```python
from build123d import *

# Parameters (mm, degrees)
BOSS_EXTRU_1_DEPTH      = 32
ESQUISSE1_7_R           = 15
BOSS_EXTRU_3_DEPTH      = 5
ESQUISSE1_8_R           = 21.5
BOSS_EXTRU_4_DEPTH      = 7
CONG_2_R                = 1
CONG_3_R                = 2.5
ESQUISSE2_R             = 2.5
ENL_V_MAT_EXTRU_1_DEPTH = 38
CONG_4_R                = 2.5
ESQUISSE3_R             = 4
ENL_V_MAT_EXTRU_2_DEPTH = 84


with BuildPart() as part:
    # Esquisse1 → Boss.-Extru.1 (new body)
    with BuildSketch(Plane.XY):
        with BuildLine():
            Line((34, -109), (34, -49))
            Line((34, -49), (54, -49))
            Line((54, -49), (54, -41))
            Line((54, -41), (34, -21))
            Line((34, -21), (34, 0))
            ThreePointArc((34, 0), (0, 34), (-34, 0))
            Line((-34, 0), (-34, -21))
            Line((-34, -21), (-54, -41))
            Line((-54, -41), (-54, -49))
            Line((-54, -49), (-34, -49))
            Line((-34, -49), (-34, -109))
            Line((-34, -109), (34, -109))
        make_face()
        with BuildLine():
            ThreePointArc((-21.5, -98.5), (-23.5, -100.5), (-25.5, -98.5))
            Line((-25.5, -98.5), (-25.5, -88.5))
            ThreePointArc((-25.5, -88.5), (-23.5, -86.5), (-21.5, -88.5))
            Line((-21.5, -88.5), (-21.5, -98.5))
        make_face(mode=Mode.SUBTRACT)
        with BuildLine():
            Line((-25.5, -51.5), (-25.5, -41.5))
            ThreePointArc((-25.5, -41.5), (-23.5, -39.5), (-21.5, -41.5))
            Line((-21.5, -41.5), (-21.5, -51.5))
            ThreePointArc((-21.5, -51.5), (-23.5, -53.5), (-25.5, -51.5))
        make_face(mode=Mode.SUBTRACT)
        with BuildLine():
            Line((25.5, -88.5), (25.5, -98.5))
            ThreePointArc((25.5, -98.5), (23.5, -100.5), (21.5, -98.5))
            Line((21.5, -98.5), (21.5, -88.5))
            ThreePointArc((21.5, -88.5), (23.5, -86.5), (25.5, -88.5))
        make_face(mode=Mode.SUBTRACT)
        with BuildLine():
            Line((21.5, -51.5), (21.5, -41.5))
            ThreePointArc((21.5, -41.5), (23.5, -39.5), (25.5, -41.5))
            Line((25.5, -41.5), (25.5, -51.5))
            ThreePointArc((25.5, -51.5), (23.5, -53.5), (21.5, -51.5))
        make_face(mode=Mode.SUBTRACT)
        with BuildLine():
            ThreePointArc((-29.608573083, -7.32), (0, 30.5), (29.608573083, -7.32))
            Line((29.608573083, -7.32), (12.1346611, -78))
            ThreePointArc((12.1346611, -78), (0, -87.5), (-12.1346611, -78))
            Line((-12.1346611, -78), (-29.608573083, -7.32))
        make_face(mode=Mode.SUBTRACT)
    extrude(amount=BOSS_EXTRU_1_DEPTH)

    # Esquisse1<7> → Boss.-Extru.3 (add)
    with BuildSketch(Plane.XY):
        with BuildLine():
            Line((34, -109), (34, -49))
            Line((34, -49), (54, -49))
            Line((54, -49), (54, -41))
            Line((54, -41), (34, -21))
            Line((34, -21), (34, 0))
            ThreePointArc((34, 0), (0, 34), (-34, 0))
            Line((-34, 0), (-34, -21))
            Line((-34, -21), (-54, -41))
            Line((-54, -41), (-54, -49))
            Line((-54, -49), (-34, -49))
            Line((-34, -49), (-34, -109))
            Line((-34, -109), (34, -109))
        make_face()
        with BuildLine():
            ThreePointArc((-21.5, -98.5), (-23.5, -100.5), (-25.5, -98.5))
            Line((-25.5, -98.5), (-25.5, -88.5))
            ThreePointArc((-25.5, -88.5), (-23.5, -86.5), (-21.5, -88.5))
            Line((-21.5, -88.5), (-21.5, -98.5))
        make_face(mode=Mode.SUBTRACT)
        with BuildLine():
            Line((-25.5, -51.5), (-25.5, -41.5))
            ThreePointArc((-25.5, -41.5), (-23.5, -39.5), (-21.5, -41.5))
            Line((-21.5, -41.5), (-21.5, -51.5))
            ThreePointArc((-21.5, -51.5), (-23.5, -53.5), (-25.5, -51.5))
        make_face(mode=Mode.SUBTRACT)
        with BuildLine():
            Line((25.5, -88.5), (25.5, -98.5))
            ThreePointArc((25.5, -98.5), (23.5, -100.5), (21.5, -98.5))
            Line((21.5, -98.5), (21.5, -88.5))
            ThreePointArc((21.5, -88.5), (23.5, -86.5), (25.5, -88.5))
        make_face(mode=Mode.SUBTRACT)
        with BuildLine():
            Line((25.5, -41.5), (25.5, -51.5))
            ThreePointArc((25.5, -51.5), (23.5, -53.5), (21.5, -51.5))
            Line((21.5, -51.5), (21.5, -41.5))
            ThreePointArc((21.5, -41.5), (23.5, -39.5), (25.5, -41.5))
        make_face(mode=Mode.SUBTRACT)
        Circle(ESQUISSE1_7_R, mode=Mode.SUBTRACT)
    extrude(amount=-BOSS_EXTRU_3_DEPTH)

    # Esquisse1<8> → Boss.-Extru.4 (add)
    with BuildSketch(Plane.XY):
        with BuildLine():
            Line((-29.608573083, -7.32), (-12.1346611, -78))
            ThreePointArc((-12.1346611, -78), (0, -87.5), (12.1346611, -78))
            Line((12.1346611, -78), (29.608573083, -7.32))
            ThreePointArc((29.608573083, -7.32), (0, 30.5), (-29.608573083, -7.32))
        make_face()
        Circle(ESQUISSE1_8_R, mode=Mode.SUBTRACT)
    extrude(amount=BOSS_EXTRU_4_DEPTH)

    # Congé2
    cong_2_edges = [part.edges().sort_by_distance(p)[0] for p in [
        (-21.5, 0, 7),
    ]]
    fillet(cong_2_edges, radius=CONG_2_R)

    # Congé3
    cong_3_edges = [part.edges().sort_by_distance(p)[0] for p in [
        (-20.871617091, -42.66, 7),
        (0, -87.5, 7),
        (20.871617091, -42.66, 7),
        (0, 30.5, 7),
    ]]
    fillet(cong_3_edges, radius=CONG_3_R)

    # Esquisse2 → Enlèv. mat.-Extru.1 (cut, through all)
    with BuildSketch(Plane(origin=(0, 0, -5), x_dir=(-1, 0, 0), z_dir=(0, 0, -1))):
        with Locations((30, -30)):
            Circle(ESQUISSE2_R)
        with Locations((-30, -30)):
            Circle(ESQUISSE2_R)
    extrude(amount=-ENL_V_MAT_EXTRU_1_DEPTH, mode=Mode.SUBTRACT)

    # Congé4
    cong_4_edges = [part.edges().sort_by_distance(p)[0] for p in [
        (34, -109, 13.5),
        (-34, -109, 13.5),
        (-34, -49, 13.5),
        (-54, -49, 13.5),
        (-54, -41, 13.5),
        (-34, -21, 13.5),
        (34, -21, 13.5),
        (54, -41, 13.5),
        (54, -49, 13.5),
        (34, -49, 13.5),
    ]]
    fillet(cong_4_edges, radius=CONG_4_R)

    # Esquisse3 → Enlèv. mat.-Extru.2 (cut, through all)
    with BuildSketch(Plane.XZ.offset(49)):
        with Locations((-44, 4)):
            Circle(ESQUISSE3_R)
        with Locations((44, 4)):
            Circle(ESQUISSE3_R)
        with Locations((44, 23)):
            Circle(ESQUISSE3_R)
        with Locations((-44, 23)):
            Circle(ESQUISSE3_R)
    extrude(amount=-ENL_V_MAT_EXTRU_2_DEPTH, mode=Mode.SUBTRACT)


solid = part.part
```
The listing builds one solid part. Answer for the finished solid, in the listing's coordinates (mm). A direction names the side the tool comes from. Coordinates: 2 decimals unless noted, no trailing zeros. Loops run counter-clockwise (first coordinate to the right, second up) from the corner with the lowest first, then second, coordinate; pieces in that order, holes last. Notation, with made-up numbers: (-3.75, -8) -> (51.25, -8) arc R26 ccw to (51.25, 8) -> close; hole circle Ø9 at (43.25, -19). An arc over 180 degrees is marked (long way). Return JSON: item names as keys, results as strings. Group by question number.
(1) Find the intervals of material crossed by probe 1 along Z at (x, y) = (44, -40.75); probe 2 along X at (y, z) = (-90, 20.5); probe 3 along Y at (x, z) = (0, -2), in increasing order. Write a range as from..to.
(2) A cutting plane is placed at C-C on x = 0. Write down the section's boundary in (y, z).
(3) Determine the mould class of faces 1 (the cylindrical face through (-40.185, -40.598, 24.201)), 2 (the flat face through (-44, -49, 14)), 3 (the cylindrical face through (-29.67, -27.52, 13.24)) for opening direction Y: released by +Y, released by -Y, zero draft, split by the parting line, or undercut.
(4) A cutting plane is placed at A-A on x = 44. Write down the section's boundary in (y, z).
(5) Given pin 1 Ø18.5 at (y, z) = (-84, 17.5) entering from -X; pin 2 Ø11 at (y, z) = (-93, 12) entering from +X; pin 3 Ø13 at (x, z) = (-44, 23) entering from +Y; pin 4 Ø7 at (x, z) = (44, 23) entering from +Y, each flat-ended and moving along its own axis, determine where each tip first touches the part or whether it passes through.
(6) A cutting plane is placed at B-B on z = 23. Count the separate pieces of the cut face and the enclosed holes in it, and give its area (3 significant figures).
(7) Which of the six approach directions +Z, -Z, +X, -X, +Y, -Y give full straight-line access (tool end or side, diameter ignored) to faces 4 (the cylindrical face through (20.26, -41.98, 7.71)), 5 (the flat face through (25.5, -93, 14)), 6 (the flat face through (34, -10, 14)), 7 (the flat face through (-16, -64, 32))?
The answers:
{
 "1": {"probe 1": "z = -5..0, 8..19, 27..32", "probe 2": "x = -34..-25.5, -21.5..21.5, 25.5..34", "probe 3": "y = -109..-15, 15..34"},
 "2": {"outline": "(-109, -5) -> (-15, -5) -> (-15, 0) -> (-21.5, 0) -> (-21.5, 6) arc R1 ccw to (-22.5, 7) -> (-85, 7) arc R2.5 cw to (-87.5, 9.5) -> (-87.5, 32) -> (-109, 32) -> close; (15, -5) -> (34, -5) -> (34, 32) -> (30.5, 32) -> (30.5, 9.5) arc R2.5 cw to (28, 7) -> (22.5, 7) arc R1 ccw to (21.5, 6) -> (21.5, 0) -> (15, 0) -> close"},
 "3": {"face 1": "zero draft", "face 2": "released by -Y", "face 3": "undercut"},
 "4": {"outline": "(-49, -5) -> (-31, -5) -> (-31, 0) -> (-49, 0) -> close; (-49, 8) -> (-31, 8) -> (-31, 19) -> (-49, 19) -> close; (-49, 27) -> (-31, 27) -> (-31, 32) -> (-49, 32) -> close"},
 "5": {"pin 1": "stops at x = -34", "pin 2": "stops at x = 34", "pin 3": "stops at y = -24.5", "pin 4": "passes through"},
 "6": {"separate pieces": "3", "enclosed holes": "7", "area": "4,380 mm^2"},
 "7": {"face 4": "+Z", "face 5": "+Z, -Z", "face 6": "+Z, -Z, +X, +Y", "face 7": "+Z, +X, -X, +Y, -Y"}
}
